from build123d import *

# Parameters (mm, degrees)
F2_W     = 101
F2_H     = 5
F3_DEPTH = 23
F4_W     = 5
F4_H     = 20
F5_DEPTH = 55.5
F1_W     = 1
F1_H     = 5
F6_DEPTH = 17.5
F7_W     = 5
F7_H     = 36
F8_DEPTH = 18.5


with BuildPart() as f3:
    # F2 (on Front) → F3 (new body, symmetric)
    with BuildSketch(Plane.XZ):
        Rectangle(F2_W, F2_H)
        Polygon((50.5, 17.5), (50.5, 2.5), (50.5, -2.5), (55.5, -2.5), (55.5, 17.5), align=None)
        Polygon((-50.5, -2.5), (-50.5, 2.5), (-50.5, 17.5), (-57.5, 17.5), (-57.5, -2.5), align=None)
    extrude(amount=F3_DEPTH, both=True)

    # F4 (on Right) → F5 (join, symmetric)
    with BuildSketch(Plane.YZ):
        with Locations((-25.5, 7.5)):
            Rectangle(F4_W, F4_H)
        with Locations((25.5, 7.5)):
            Rectangle(F4_W, F4_H)
    extrude(amount=F5_DEPTH, both=True)

    # F1 (on Top) → F6 (join)
    with BuildSketch(Plane.XY):
        with Locations((-50, 20.5)):
            Rectangle(F1_W, F1_H)
        with Locations((-45, 20.5)):
            Rectangle(F1_W, F1_H)
        with Locations((-40, 20.5)):
            Rectangle(F1_W, F1_H)
        with Locations((-35, 20.5)):
            Rectangle(F1_W, F1_H)
        with Locations((-30, 20.5)):
            Rectangle(F1_W, F1_H)
        with Locations((-25, 20.5)):
            Rectangle(F1_W, F1_H)
        with Locations((-20, 20.5)):
            Rectangle(F1_W, F1_H)
        with Locations((-15, 20.5)):
            Rectangle(F1_W, F1_H)
        with Locations((-10, 20.5)):
            Rectangle(F1_W, F1_H)
        with Locations((-5, 20.5)):
            Rectangle(F1_W, F1_H)
        with Locations((0, 20.5)):
            Rectangle(F1_W, F1_H)
        with Locations((5, 20.5)):
            Rectangle(F1_W, F1_H)
        with Locations((10, 20.5)):
            Rectangle(F1_W, F1_H)
        with Locations((15, 20.5)):
            Rectangle(F1_W, F1_H)
        with Locations((20, 20.5)):
            Rectangle(F1_W, F1_H)
        with Locations((25, 20.5)):
            Rectangle(F1_W, F1_H)
        with Locations((30, 20.5)):
            Rectangle(F1_W, F1_H)
        with Locations((35, 20.5)):
            Rectangle(F1_W, F1_H)
        with Locations((40, 20.5)):
            Rectangle(F1_W, F1_H)
        with Locations((45, 20.5)):
            Rectangle(F1_W, F1_H)
        with Locations((50, 20.5)):
            Rectangle(F1_W, F1_H)
        with Locations((-50, -20.5)):
            Rectangle(F1_W, F1_H)
        with Locations((50, -20.5)):
            Rectangle(F1_W, F1_H)
        with Locations((-45, -20.5)):
            Rectangle(F1_W, F1_H)
        with Locations((0, -20.5)):
            Rectangle(F1_W, F1_H)
        with Locations((20, -20.5)):
            Rectangle(F1_W, F1_H)
        with Locations((40, -20.5)):
            Rectangle(F1_W, F1_H)
        with Locations((-20, -20.5)):
            Rectangle(F1_W, F1_H)
        with Locations((30, -20.5)):
            Rectangle(F1_W, F1_H)
        with Locations((-35, -20.5)):
            Rectangle(F1_W, F1_H)
        with Locations((-30, -20.5)):
            Rectangle(F1_W, F1_H)
        with Locations((-10, -20.5)):
            Rectangle(F1_W, F1_H)
        with Locations((10, -20.5)):
            Rectangle(F1_W, F1_H)
        with Locations((-40, -20.5)):
            Rectangle(F1_W, F1_H)
        with Locations((35, -20.5)):
            Rectangle(F1_W, F1_H)
        with Locations((-25, -20.5)):
            Rectangle(F1_W, F1_H)
        with Locations((-5, -20.5)):
            Rectangle(F1_W, F1_H)
        with Locations((15, -20.5)):
            Rectangle(F1_W, F1_H)
        with Locations((5, -20.5)):
            Rectangle(F1_W, F1_H)
        with Locations((25, -20.5)):
            Rectangle(F1_W, F1_H)
        with Locations((45, -20.5)):
            Rectangle(F1_W, F1_H)
        with Locations((-15, -20.5)):
            Rectangle(F1_W, F1_H)
    extrude(amount=F6_DEPTH)

    # F7 (on Top) → F8 (join)
    with BuildSketch(Plane.XY):
        with Locations((-54, 0.467316)):
            Rectangle(F7_W, F7_H)
    extrude(amount=F8_DEPTH)


solid = f3.part
Input: part model. Units: mm. Frame: model coordinates. A direction names the side the tool comes from. Round coordinates to 2 decimals unless told otherwise and drop trailing zeros. Write each loop counter-clockwise with the first axis right and the second up, starting at its lowest first coordinate (ties: lowest second). Pieces come first, ordered by that corner, then holes.
1) Cut plane B-B (x = 37.5). Return the cut outline in (y, z), then the cut area to 3 significant figures.
2) Contact query for a flat-ended pin moving along its axis: P1, Ø2, axis at x = -39, y = 13, coming from the +Z side. Output: stop coordinate, or through.
3) Cut plane A-A (y = -6.5). Return the cut outline in (x, z), then the cut area to 3 significant figures.
4) Ray query, L1, parallel to X at y = -7, z = 17; L2, parallel to Y at x = -27.5, z = 14; L3, parallel to Z at x = -24, y = 13.5. Return the intervals inside material, ascending.
5) Draft query along Y for faces 1 (the flat face through (-57, -23, 8)), 2 (the flat face through (-32, 23, 10)), 3 (the flat face through (55.5, 0, 8)). Return one class per face: pulls with the +Y half, pulls with the -Y half, needs draft (parallel to the pull), parting line crosses it, or undercut.
6) Cut plane C-C (y = 24.5). Return the cut outline in (x, z), then the cut area to 3 significant figures.
7) Reachability of faces 4 (the flat face through (44.5, -21, 10)), 5 (the flat face through (-57.5, 0, 8)) from +Z, -Z, +X, -X, +Y, -Y: full face, straight path, thin tool, end or side. Return the list, or none.
Geometry says:
1. outline: (-28, -2.5) - (28, -2.5) - (28, 17.5) - (23, 17.5) - (23, 2.5) - (-23, 2.5) - (-23, 17.5) - (-28, 17.5) - close
1. area: 430 mm2
2. P1: stops at z = 2.5
3. outline: (-57.5, -2.5) - (55.5, -2.5) - (55.5, 17.5) - (50.5, 17.5) - (50.5, 2.5) - (-50.5, 2.5) - (-50.5, 17.5) - (-51.5, 17.5) - (-51.5, 18.5) - (-56.5, 18.5) - (-56.5, 17.5) - (-57.5, 17.5) - close
3. area: 750 mm2
4. L1: x = -57.5 to -50.5, 50.5 to 55.5
4. L2: y = -28 to -23, 23 to 28
4. L3: z = -2.5 to 2.5
5. face 1: pulls with the -Y half
5. face 2: undercut
5. face 3: needs draft
6. outline: (-55.5, -2.5) - (55.5, -2.5) - (55.5, 17.5) - (-55.5, 17.5) - close
6. area: 2,220 mm2
7. face 4: +Z
7. face 5: +Z, -Z, -X, +Y, -Y
